Input: part model. Units: mm. Frame: model coordinates. Face numbers are marked on the shaded views. A direction names the side the tool comes from. Coordinates: 2 decimals unless noted, no trailing zeros. Loops run counter-clockwise (first coordinate to the right, second up) from the corner with the lowest first, then second, coordinate; pieces in that order, holes last.
Autodesk Inventor part; units mm, degrees
ref_plane "YZ Plane" through (0, 0, 0) normal (1, 0, 0) x (0, 1, 0)
ref_plane "XZ Plane" through (0, 0, 0) normal (0, 1, 0) x (-1, 0, 0)
ref_plane "XY Plane" through (0, 0, 0) normal (0, 0, 1) x (1, 0, 0)
sketch "Sketch1" plane through (0, 0, 0) normal (0, 0, 1) x (1, 0, 0)
  circle A0 centre (-414.4261, -56.251) radius 4.7625
  point P0 (0, 0)
  dimension "d0" = 9.525
extrude "Extrusion1" add sketch "Sketch1" against normal blind 139.7
sketch "Sketch2" plane through (-414.4261, -56.251, 0) normal (0, 0, 1) x (1, 0, 0)
  circle A0 centre (0, 0) radius 4.7625
  line L0 (-8.2489, 0) -> (-4.1244, 7.1437)
  line L1 (-4.1244, 7.1437) -> (4.1244, 7.1438)
  line L2 (4.1244, 7.1438) -> (8.2489, 0)
  line L3 (8.2489, 0) -> (4.1244, -7.1437)
  line L4 (4.1244, -7.1437) -> (-4.1244, -7.1438)
  line L5 (-4.1244, -7.1438) -> (-8.2489, 0)
  point P0 (414.4261, 56.251)
  dimension "d3" = 14.2875
extrude "Extrusion2" add sketch "Sketch2" along normal blind 3.175 contours A0 | L0 L1 L2 L3 L4 L5
thread "Thread1"
chamfer "Chamfer1" distance 0.508 angle 45 1 edges at (-419.1886, -56.251, -139.7)
properties part number "375 bolt x4" material "Steel"
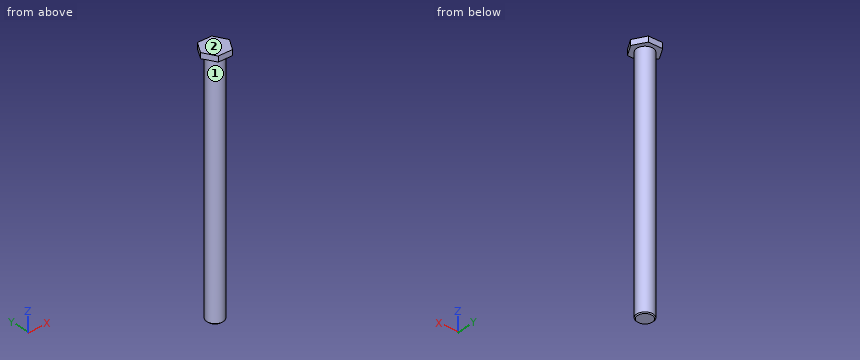
Item 1: Line query: L1, parallel to Z at x = -410.5, y = -50 (3 decimals); L2, parallel to Y at x = -414.5, z = -128; L3, parallel to X at y = -57.25, z = -114.5. Output: solid intervals per line, ascending.
Result:
L1: z = 0 to 3.175
L2: y = -61.01 to -51.49
L3: x = -419.08 to -409.77
Item 2: Contact query for flat-ended pins moving along their axis: P1, Ø3, axis at y = -58.5, z = -104.5, coming from the -X side; P2, Ø6, axis at x = -408, z = -101, coming from the -Y side; P3, Ø1, axis at x = -416, z = -33.5, coming from the -Y side. Output: stop coordinate, or through.
Result:
P1: stops at x = -419.13
P2: stops at y = -59.56
P3: stops at y = -60.89
Item 3: Section query C-C (x = -408.5). Output: boundary loops of the cut face in (y, z) (3 decimals).
Result:
outline: (-60.274, 0) - (-52.228, 0) - (-52.228, 3.175) - (-60.274, 3.175) - close
Item 4: Section query B-B (x = -421). Output: boundary loops of the cut face in (y, z) (3 decimals).
Result:
outline: (-59.152, 0) - (-53.35, 0) - (-53.35, 3.175) - (-59.152, 3.175) - close
Item 5: Reachability of the marked faces 1 and 2 from +Z, -Z, +X, -X, +Y, -Y: full face, straight path, thin tool, end or side. Return the list, or none.
Result:
face 1: -Z
face 2: +Z, +X, -X, +Y, -Y
Item 6: Section query A-A (z = -91). Output: boundary loops of the cut face in (x, y) (1 decimal).
Result:
outline: circle Ø9.5 at (-414.4, -56.3)
